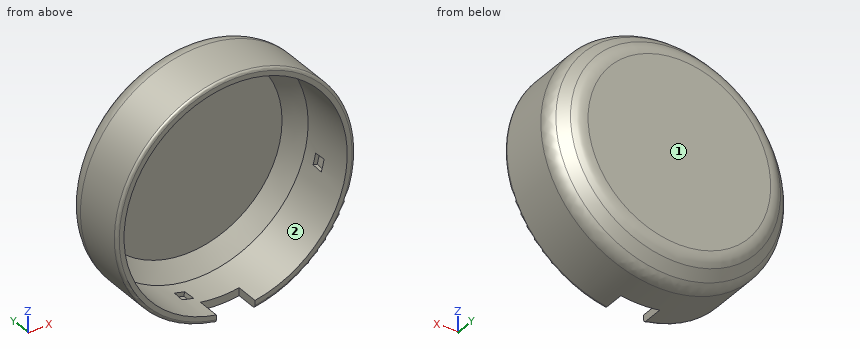
```python
from build123d import *

# Parameters (mm, degrees)
SKETCH1_R           = 14.6431
BOSS_EXTRUDE1_DEPTH = 9.525
FILLET1_SIZE        = 2.032
SHELL1_T            = 1.016
SKETCH2_W           = 5.08
SKETCH2_H           = 3.048
CUT_EXTRUDE1_DEPTH  = 25.4
FILLET2_R           = 0.381
SNAP_START          = -15.1892
SNAP_GROOVE1_DEPTH  = 0.567483728
CIRPATTERN2_COUNT   = 4
FILLET3_R           = 2.54
FILLET4_R           = 2.54


# Read off the part's stored shape, not the designer's step: Snap Groove1
with BuildPart() as part:
    # Sketch1 → Boss-Extrude1 (new body)
    with BuildSketch(Plane(origin=(0, 0, 0), x_dir=(1, 0, 0), z_dir=(0, 1, 0))):
        with Locations(Location((0, 0, 0), (0, 0, 90))):
            Circle(SKETCH1_R)
    extrude(amount=BOSS_EXTRUDE1_DEPTH)

    # Fillet1
    fillet1_edges = [part.edges().sort_by_distance(p)[0] for p in [
        (0, 9.525, 14.6431),
    ]]
    chamfer(fillet1_edges, length=FILLET1_SIZE)

    # Shell1
    shell1_openings = [part.faces().sort_by_distance(p)[0] for p in [
        (0, 0, 0),
    ]]
    offset(amount=SHELL1_T, openings=shell1_openings, kind=Kind.INTERSECTION)

    # Sketch2 → Cut-Extrude1 (cut)
    with BuildSketch(Plane.XY):
        with Locations((0, 1.524)):
            Rectangle(SKETCH2_W, SKETCH2_H)
    extrude(amount=-CUT_EXTRUDE1_DEPTH, mode=Mode.SUBTRACT)

    # Fillet2
    fillet2_edges = [part.edges().sort_by_distance(p)[0] for p in [
        (0, 0, 15.6591),
    ]]
    fillet(fillet2_edges, radius=FILLET2_R)

    # Snap Groove1 outline → Snap Groove1 (cut)
    with BuildSketch(Plane(origin=(0, 0, 0), x_dir=(0.9711506345911166, 0, -0.23846686338623996), z_dir=(0.23846686338623993, 0, 0.9711506345911166)).offset(SNAP_START)):
        Polygon((-0.707206527, 5.6642), (-0.791069456, 4.064), (0.791069456, 4.064), (0.707206527, 5.6642), align=None)
    snap_groove1 = extrude(amount=SNAP_GROOVE1_DEPTH, mode=Mode.SUBTRACT)

    # CirPattern2: Snap Groove1 ×4 about axis
    cirpattern2_axis = Axis((0, 0, 0), (0, 1, 0))
    for i in range(1, CIRPATTERN2_COUNT):
        add(snap_groove1.rotate(cirpattern2_axis, i * 360 / CIRPATTERN2_COUNT), mode=Mode.SUBTRACT)

    # Fillet3
    fillet3_edges = [part.edges().sort_by_distance(p)[0] for p in [
        (0, 7.913840979, 15.6591),
    ]]
    fillet(fillet3_edges, radius=FILLET3_R)

    # Fillet4
    fillet4_edges = [part.edges().sort_by_distance(p)[0] for p in [
        (0, 10.541, 13.031940979),
    ]]
    fillet(fillet4_edges, radius=FILLET4_R)


solid = part.part
```
For this review, take the finished solid that the model builds, in its own axes (mm). Face numbers are marked on the shaded views. A direction names the side the tool comes from. Coordinates: 2 decimals unless noted, no trailing zeros. Write each loop counter-clockwise with the first axis right and the second up, starting at its lowest first coordinate (ties: lowest second). Pieces come first, ordered by that corner, then holes. Notation, with made-up numbers: (-11, 7.5) - (42, 7.5) arc R17 ccw to (42, 35.5) - close; hole circle Ø11 at (37.5, 16). An arc over 180 degrees is marked (long way). Answer in a Markdown table with one row per item. Add a question column.
Q1. For probe 1 along X at (y, z) = (5.75, 0); probe 2 along Z at (x, y) = (8, 2.5); probe 3 along Z at (x, y) = (1, 8.75), list the stretches that pass through material, from the lowest coordinate up.
Q2. Tool access review of the marked faces 1 and 2: name each direction out of +Z, -Z, +X, -X, +Y, -Y from which nothing blocks a thin tool from reaching the whole face with its end or side.
Q3. We need section A-A, the plane y = 5. State the section outline as (x, z) points.
Q4. For P1, Ø1.1, axis at y = 1, z = -15, coming from the -X side; P2, Ø3, axis at x = 0, z = 8.5, coming from the -Y side (3 decimals); P3, Ø2, axis at x = -3.5, y = 5.5, coming from the -Z side, all flat-tipped, find the tip position at first contact; note any pin that passes through.
Answer list:
| question | item | result |
|---|---|---|
| 1 | probe 1 | x = -15.66 to -14.64, 14.64 to 15.66 |
| 1 | probe 2 | z = -13.46 to -12.26, 12.26 to 13.46 |
| 1 | probe 3 | z = -14.79 to -13.35, 13.35 to 14.79 |
| 2 | face 1 | +Z, -Z, +X, -X, +Y |
| 2 | face 2 | -Y |
| 3 | outline | circle Ø31.32 at (0, 0); hole (-14.93, 2.9) - (-14.38, 2.77) arc R14.64 ccw to (-4.21, -14.03) - (-4.34, -14.57) - (-2.9, -14.93) - (-2.77, -14.38) arc R14.64 ccw to (14.03, -4.21) - (14.57, -4.34) - (14.93, -2.9) - (14.38, -2.77) arc R14.64 ccw to (4.21, 14.03) - (4.34, 14.57) - (2.9, 14.93) - (2.77, 14.38) arc R14.64 ccw to (-14.03, 4.21) - (-14.57, 4.34) - close |
| 4 | P1 | stops at x = -6.03 |
| 4 | P2 | stops at y = 9.525 |
| 4 | P3 | stops at z = -15.46 |
